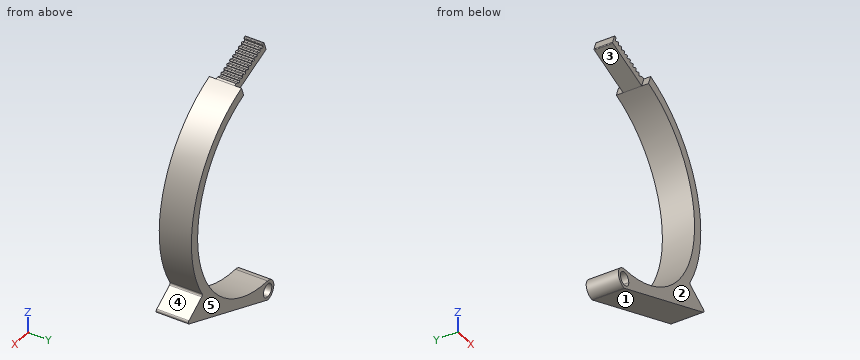
from build123d import *

# Parameters (mm, degrees)
BOSS_EXTRUDE1_DEPTH = 13
CUT_EXTRUDE1_DEPTH  = 20
FILLET2_R           = 0.3
FILLET1_R           = 0.8
SKETCH3_OUTSIDE_W   = 144.199
SKETCH3_OUTSIDE_H   = 38.986
SKETCH3_OUTSIDE_W_2 = 5.910380326
SKETCH3_OUTSIDE_H_2 = 7.5
CUT_EXTRUDE2_DEPTH  = 20


with BuildPart() as part:
    # Sketch1 → Boss-Extrude1 (new body)
    with BuildSketch(Plane(origin=(0, 0, 0), x_dir=(1, 0, 0), z_dir=(0, 1, 0))):
        with BuildLine():
            Line((0, 51.7), (0, 53))
            ThreePointArc((0, 53), (-4, 49), (0, 45))
            ThreePointArc((0, 45), (44.316348886, 7.814167995), (15.39090645, -42.286167935))
            Line((15.39090645, -42.286167935), (-3.402945966, -49.126570802))
            Line((-3.402945966, -49.126570802), (-2.034865393, -52.885341285))
            Line((-2.034865393, -52.885341285), (16.758987023, -46.044938419))
            ThreePointArc((16.758987023, -46.044938419), (46.283080581, -16.089638031), (41.707047143, 25.720074234))
            ThreePointArc((41.707047143, 25.720074234), (25.051905135, 42.111780407), (2.698975076, 48.925612245))
            ThreePointArc((2.698975076, 48.925612245), (-1.935309657, 47.117295421), (0, 51.7))
        make_face()
        with BuildLine():
            Line((51.921017872, 32.018867925), (0, 53))
            Line((0, 53), (0, 51.7))
            ThreePointArc((0, 51.7), (1.909188309, 50.909188309), (2.7, 49))
            ThreePointArc((2.7, 49), (2.699743757, 48.962802592), (2.698975076, 48.925612245))
            ThreePointArc((2.698975076, 48.925612245), (25.051905135, 42.111780407), (41.707047143, 25.720074234))
            Line((41.707047143, 25.720074234), (51.921017872, 32.018867925))
        make_face()
    extrude(amount=BOSS_EXTRUDE1_DEPTH)

    # Sketch2 → Cut-Extrude1 (cut)
    with BuildSketch(Plane(origin=(0, 13, 0), x_dir=(1, 0, 0), z_dir=(0, 1, 0))):
        Polygon((-1.71080903, -50.851874424), (-1.095172772, -52.543321142), (0.78421247, -51.859280855), align=None)
        Polygon((0.168576212, -50.167834138), (0.78421247, -51.859280855), (2.663597711, -51.175240568), align=None)
        Polygon((2.047961453, -49.483793851), (2.663597711, -51.175240568), (4.542982953, -50.491200282), align=None)
        Polygon((3.927346695, -48.799753564), (4.542982953, -50.491200282), (6.422368194, -49.807159995), align=None)
        Polygon((5.806731936, -48.115713278), (6.422368194, -49.807159995), (8.301753436, -49.123119708), align=None)
        Polygon((7.686117178, -47.431672991), (8.301753436, -49.123119708), (10.181138677, -48.439079422), align=None)
        Polygon((9.565502419, -46.747632704), (10.181138677, -48.439079422), (12.060523919, -47.755039135), align=None)
        Polygon((11.444887661, -46.063592418), (12.060523919, -47.755039135), (13.939909161, -47.070998848), align=None)
        Polygon((13.324272903, -45.379552131), (13.939909161, -47.070998848), (15.819294402, -46.386958562), align=None)
    extrude(amount=-CUT_EXTRUDE1_DEPTH, mode=Mode.SUBTRACT)

    # Fillet2
    fillet2_edges = [part.edges().sort_by_distance(p)[0] for p in [
        (0.168576212, 6.5, 50.167834138),
        (3.927346695, 6.5, 48.799753564),
        (7.686117178, 6.5, 47.431672991),
        (11.444887661, 6.5, 46.063592418),
        (-2.034865393, 6.5, 52.885341285),
        (-3.402945966, 6.5, 49.126570802),
        (-1.71080903, 6.5, 50.851874424),
        (0.78421247, 6.5, 51.859280855),
        (-1.095172772, 6.5, 52.543321142),
        (2.047961453, 6.5, 49.483793851),
        (4.542982953, 6.5, 50.491200282),
        (2.663597711, 6.5, 51.175240568),
        (5.806731936, 6.5, 48.115713278),
        (8.301753436, 6.5, 49.123119708),
        (6.422368194, 6.5, 49.807159995),
        (9.565502419, 6.5, 46.747632704),
        (12.060523919, 6.5, 47.755039135),
        (10.181138677, 6.5, 48.439079422),
        (13.324272903, 6.5, 45.379552131),
        (15.819294402, 6.5, 46.386958562),
        (13.939909161, 6.5, 47.070998848),
    ]]
    fillet(fillet2_edges, radius=FILLET2_R)

    # Fillet1
    fillet1_edges = [part.edges().sort_by_distance(p)[0] for p in [
        (51.921017872, 6.5, -32.018867925),
        (41.707047143, 6.5, -25.720074234),
        (0, 6.5, -53),
    ]]
    fillet(fillet1_edges, radius=FILLET1_R)

    # Sketch3 outside → Cut-Extrude2 (cut)
    with BuildSketch(Plane(origin=(-18.793852416, 0, 6.840402867), x_dir=(0.342020143, 0, 0.939692621), z_dir=(-0.939692621, 0, 0.342020143))):
        with Locations((7.9375, 6.5)):
            Rectangle(SKETCH3_OUTSIDE_W, SKETCH3_OUTSIDE_H)
        with Locations((47.141631591, 6.5)):
            Rectangle(SKETCH3_OUTSIDE_W_2, SKETCH3_OUTSIDE_H_2, mode=Mode.SUBTRACT)
    extrude(amount=-CUT_EXTRUDE2_DEPTH, mode=Mode.SUBTRACT)


solid = part.part
Work out the finished part from the listing and answer in its coordinate system (mm). Face numbers are marked on the shaded views. A direction names the side the tool comes from. Coordinates: 2 decimals unless noted, no trailing zeros. Write each loop counter-clockwise with the first axis right and the second up, starting at its lowest first coordinate (ties: lowest second). Pieces come first, ordered by that corner, then holes.
1. For a pull along Z with two mould halves and no side action, classify the marked faces 1, 2 and 3 as +Z half, -Z half, draft (parallel to the pull), parting line (faces both ways), or undercut.
Results list:
face 1: -Z half
face 2: draft
face 3: undercut
2. For the marked faces 4 and 5, determine the directions among +Z, -Z, +X, -X, +Y, -Y from which every point of the face is accessible in a straight line to the end or side of a thin tool.
Results list:
face 4: +X, +Y, -Y
face 5: +Z, -Z, +X, -X, +Y
3. The part is cut by section A-A, the plane x = 36.5. Write down the section's boundary in (y, z), and give its area (3 significant figures).
Results list:
outline: (0, -38.25) - (13, -38.25) - (13, -26.32) - (0, -26.32) - close; (0, 26.32) - (13, 26.32) - (13, 32.69) - (0, 32.69) - close
area: 238 mm2
4. Consider line 1 along Z through (x, y) = (0, 8); line 2 along Z through (x, y) = (20, 9.25); line 3 along Z through (x, y) = (29, 2). Determine where each line is inside the solid, lowest interval first.
Results list:
line 1: z = -52.98 to -51.7, -46.3 to -45, 47.89 to 51.54
line 2: z = -44.92 to -40.31, 40.31 to 44.73
line 3: z = -41.28 to -34.41, 34.41 to 39.5
5. The part is cut by section B-B, the plane z = 44. Write down the section's boundary in (x, y), and give its area (3 significant figures).
Results list:
outline: (10.68, 2.75) - (16.01, 2.75) - (16.01, 0) - (21.56, 0) - (21.56, 13) - (16.01, 13) - (16.01, 10.25) - (10.68, 10.25) - close
area: 112 mm2
6. The part is cut by section D-D, the plane z = -1. Write down the section's boundary in (x, y).
Results list:
outline: (44.99, 0) - (48.99, 0) - (48.99, 13) - (44.99, 13) - close
7. Flat-ended cylindrical pins translate along their axes: pin 1 (2 mm diameter, centred on x = 12.5, y = 2, fed in from -Z); pin 2 (6 mm diameter, centred on x = 34.5, y = 1.5, fed in from -Z); pin 3 (8.5 mm diameter, centred on x = 6.5, z = 49, fed in from +Y); pin 4 (7 mm diameter, centred on x = 0, z = -49, fed in from -Y). Find the tip coordinate at first contact, or state that the pin passes through.
Results list:
pin 1: stops at z = -48.35
pin 2: stops at z = -40.27
pin 3: stops at y = 10.25
pin 4: stops at y = 0
8. The part is cut by section C-C, the plane x = 28.5. Write down the section's boundary in (y, z).
Results list:
outline: (0, -41.48) - (13, -41.48) - (13, -34.82) - (0, -34.82) - close; (0, 34.82) - (13, 34.82) - (13, 39.86) - (0, 39.86) - close
